```python
from build123d import *

# Parameters (mm, degrees)
SKETCH1_R           = 1.5
BOSS_EXTRUDE1_DEPTH = 3
FILLET1_R           = 0.5


with BuildPart() as part:
    # Sketch1 → Boss-Extrude1 (new body)
    with BuildSketch(Plane.XY):
        with BuildLine():
            ThreePointArc((31, -4), (35, 0), (31, 4))
            Line((31, 4), (11.967993881, 4))
            ThreePointArc((11.967993881, 4), (12.864888434, 4.573115684), (13.63194632, 5.311020574))
            ThreePointArc((13.63194632, 5.311020574), (13.516357561, 5.598658616), (13.394700346, 5.883783021))
            ThreePointArc((13.394700346, 5.883783021), (12.067442445, 5.825370588), (10.794615193, 5.444665539))
            ThreePointArc((10.794615193, 5.444665539), (10.470247132, 6.045), (10.112526268, 6.626078212))
            ThreePointArc((10.112526268, 6.626078212), (11.078640138, 7.538026423), (11.79285574, 8.658259265))
            ThreePointArc((11.79285574, 8.658259265), (11.606759368, 8.906179706), (11.415451897, 9.150101529))
            ThreePointArc((11.415451897, 9.150101529), (10.148537462, 8.750159829), (9.017614465, 8.052995056))
            ThreePointArc((9.017614465, 8.052995056), (8.548920985, 8.548920985), (8.052995056, 9.017614465))
            ThreePointArc((8.052995056, 9.017614465), (8.750159829, 10.148537462), (9.150101529, 11.415451897))
            ThreePointArc((9.150101529, 11.415451897), (8.906179706, 11.606759368), (8.658259265, 11.79285574))
            ThreePointArc((8.658259265, 11.79285574), (7.538026423, 11.078640138), (6.626078212, 10.112526268))
            ThreePointArc((6.626078212, 10.112526268), (6.045, 10.470247132), (5.444665539, 10.794615193))
            ThreePointArc((5.444665539, 10.794615193), (5.825370588, 12.067442445), (5.883783021, 13.394700346))
            ThreePointArc((5.883783021, 13.394700346), (5.598658616, 13.516357561), (5.311020574, 13.63194632))
            ThreePointArc((5.311020574, 13.63194632), (4.413811339, 12.65212943), (3.78298568, 11.482905527))
            ThreePointArc((3.78298568, 11.482905527), (3.129122255, 11.67804324), (2.465291063, 11.835980736))
            ThreePointArc((2.465291063, 11.835980736), (2.503591968, 13.163971168), (2.216494423, 14.461122103))
            ThreePointArc((2.216494423, 14.461122103), (1.909598192, 14.504838322), (1.601844607, 14.542042286))
            ThreePointArc((1.601844607, 14.542042286), (0.988802307, 13.36339701), (0.682088925, 12.070743751))
            ThreePointArc((0.682088925, 12.070743751), (0, 12.09), (-0.682088925, 12.070743751))
            ThreePointArc((-0.682088925, 12.070743751), (-0.988802307, 13.36339701), (-1.601844607, 14.542042286))
            ThreePointArc((-1.601844607, 14.542042286), (-1.909598192, 14.504838322), (-2.216494423, 14.461122103))
            ThreePointArc((-2.216494423, 14.461122103), (-2.503591968, 13.163971168), (-2.465291063, 11.835980736))
            ThreePointArc((-2.465291063, 11.835980736), (-3.129122255, 11.67804324), (-3.78298568, 11.482905527))
            ThreePointArc((-3.78298568, 11.482905527), (-4.413811339, 12.65212943), (-5.311020574, 13.63194632))
            ThreePointArc((-5.311020574, 13.63194632), (-5.598658616, 13.516357561), (-5.883783021, 13.394700346))
            ThreePointArc((-5.883783021, 13.394700346), (-5.825370588, 12.067442445), (-5.444665539, 10.794615193))
            ThreePointArc((-5.444665539, 10.794615193), (-6.045, 10.470247132), (-6.626078212, 10.112526268))
            ThreePointArc((-6.626078212, 10.112526268), (-7.538026423, 11.078640138), (-8.658259265, 11.79285574))
            ThreePointArc((-8.658259265, 11.79285574), (-8.906179706, 11.606759368), (-9.150101529, 11.415451897))
            ThreePointArc((-9.150101529, 11.415451897), (-8.750159829, 10.148537462), (-8.052995056, 9.017614465))
            ThreePointArc((-8.052995056, 9.017614465), (-8.548920985, 8.548920985), (-9.017614465, 8.052995056))
            ThreePointArc((-9.017614465, 8.052995056), (-10.148537462, 8.750159829), (-11.415451897, 9.150101529))
            ThreePointArc((-11.415451897, 9.150101529), (-11.606759368, 8.906179706), (-11.79285574, 8.658259265))
            ThreePointArc((-11.79285574, 8.658259265), (-11.078640138, 7.538026423), (-10.112526268, 6.626078212))
            ThreePointArc((-10.112526268, 6.626078212), (-10.470247132, 6.045), (-10.794615193, 5.444665539))
            ThreePointArc((-10.794615193, 5.444665539), (-12.067442445, 5.825370588), (-13.394700346, 5.883783021))
            ThreePointArc((-13.394700346, 5.883783021), (-13.516357561, 5.598658616), (-13.63194632, 5.311020574))
            ThreePointArc((-13.63194632, 5.311020574), (-12.65212943, 4.413811339), (-11.482905527, 3.78298568))
            ThreePointArc((-11.482905527, 3.78298568), (-11.67804324, 3.129122255), (-11.835980736, 2.465291063))
            ThreePointArc((-11.835980736, 2.465291063), (-13.163971168, 2.503591968), (-14.461122103, 2.216494423))
            ThreePointArc((-14.461122103, 2.216494423), (-14.504838322, 1.909598192), (-14.542042286, 1.601844607))
            ThreePointArc((-14.542042286, 1.601844607), (-13.36339701, 0.988802307), (-12.070743751, 0.682088925))
            ThreePointArc((-12.070743751, 0.682088925), (-12.09, 0), (-12.070743751, -0.682088925))
            ThreePointArc((-12.070743751, -0.682088925), (-13.36339701, -0.988802307), (-14.542042286, -1.601844607))
            ThreePointArc((-14.542042286, -1.601844607), (-14.504838322, -1.909598192), (-14.461122103, -2.216494423))
            ThreePointArc((-14.461122103, -2.216494423), (-13.163971168, -2.503591968), (-11.835980736, -2.465291063))
            ThreePointArc((-11.835980736, -2.465291063), (-11.67804324, -3.129122255), (-11.482905527, -3.78298568))
            ThreePointArc((-11.482905527, -3.78298568), (-12.65212943, -4.413811339), (-13.63194632, -5.311020574))
            ThreePointArc((-13.63194632, -5.311020574), (-13.516357561, -5.598658616), (-13.394700346, -5.883783021))
            ThreePointArc((-13.394700346, -5.883783021), (-12.067442445, -5.825370588), (-10.794615193, -5.444665539))
            ThreePointArc((-10.794615193, -5.444665539), (-10.470247132, -6.045), (-10.112526268, -6.626078212))
            ThreePointArc((-10.112526268, -6.626078212), (-11.078640138, -7.538026423), (-11.79285574, -8.658259265))
            ThreePointArc((-11.79285574, -8.658259265), (-11.606759368, -8.906179706), (-11.415451897, -9.150101529))
            ThreePointArc((-11.415451897, -9.150101529), (-10.148537462, -8.750159829), (-9.017614465, -8.052995056))
            ThreePointArc((-9.017614465, -8.052995056), (-8.548920985, -8.548920985), (-8.052995056, -9.017614465))
            ThreePointArc((-8.052995056, -9.017614465), (-8.750159829, -10.148537462), (-9.150101529, -11.415451897))
            ThreePointArc((-9.150101529, -11.415451897), (-8.906179706, -11.606759368), (-8.658259265, -11.79285574))
            ThreePointArc((-8.658259265, -11.79285574), (-7.538026423, -11.078640138), (-6.626078212, -10.112526268))
            ThreePointArc((-6.626078212, -10.112526268), (-6.045, -10.470247132), (-5.444665539, -10.794615193))
            ThreePointArc((-5.444665539, -10.794615193), (-5.825370588, -12.067442445), (-5.883783021, -13.394700346))
            ThreePointArc((-5.883783021, -13.394700346), (-5.598658616, -13.516357561), (-5.311020574, -13.63194632))
            ThreePointArc((-5.311020574, -13.63194632), (-4.413811339, -12.65212943), (-3.78298568, -11.482905527))
            ThreePointArc((-3.78298568, -11.482905527), (-3.129122255, -11.67804324), (-2.465291063, -11.835980736))
            ThreePointArc((-2.465291063, -11.835980736), (-2.503591968, -13.163971168), (-2.216494423, -14.461122103))
            ThreePointArc((-2.216494423, -14.461122103), (-1.909598192, -14.504838322), (-1.601844607, -14.542042286))
            ThreePointArc((-1.601844607, -14.542042286), (-0.988802307, -13.36339701), (-0.682088925, -12.070743751))
            ThreePointArc((-0.682088925, -12.070743751), (0, -12.09), (0.682088925, -12.070743751))
            ThreePointArc((0.682088925, -12.070743751), (0.988802307, -13.36339701), (1.601844607, -14.542042286))
            ThreePointArc((1.601844607, -14.542042286), (1.909598192, -14.504838322), (2.216494423, -14.461122103))
            ThreePointArc((2.216494423, -14.461122103), (2.503591968, -13.163971168), (2.465291063, -11.835980736))
            ThreePointArc((2.465291063, -11.835980736), (3.129122255, -11.67804324), (3.78298568, -11.482905527))
            ThreePointArc((3.78298568, -11.482905527), (4.413811339, -12.65212943), (5.311020574, -13.63194632))
            ThreePointArc((5.311020574, -13.63194632), (5.598658616, -13.516357561), (5.883783021, -13.394700346))
            ThreePointArc((5.883783021, -13.394700346), (5.825370588, -12.067442445), (5.444665539, -10.794615193))
            ThreePointArc((5.444665539, -10.794615193), (6.045, -10.470247132), (6.626078212, -10.112526268))
            ThreePointArc((6.626078212, -10.112526268), (7.538026423, -11.078640138), (8.658259265, -11.79285574))
            ThreePointArc((8.658259265, -11.79285574), (8.906179706, -11.606759368), (9.150101529, -11.415451897))
            ThreePointArc((9.150101529, -11.415451897), (8.750159829, -10.148537462), (8.052995056, -9.017614465))
            ThreePointArc((8.052995056, -9.017614465), (8.548920985, -8.548920985), (9.017614465, -8.052995056))
            ThreePointArc((9.017614465, -8.052995056), (10.148537462, -8.750159829), (11.415451897, -9.150101529))
            ThreePointArc((11.415451897, -9.150101529), (11.606759368, -8.906179706), (11.79285574, -8.658259265))
            ThreePointArc((11.79285574, -8.658259265), (11.078640138, -7.538026423), (10.112526268, -6.626078212))
            ThreePointArc((10.112526268, -6.626078212), (10.470247132, -6.045), (10.794615193, -5.444665539))
            ThreePointArc((10.794615193, -5.444665539), (12.067442445, -5.825370588), (13.394700346, -5.883783021))
            ThreePointArc((13.394700346, -5.883783021), (13.516357561, -5.598658616), (13.63194632, -5.311020574))
            ThreePointArc((13.63194632, -5.311020574), (12.864888434, -4.573115684), (11.967993881, -4))
            Line((11.967993881, -4), (31, -4))
        make_face()
        Circle(SKETCH1_R, mode=Mode.SUBTRACT)
        with Locations((31, 0)):
            Circle(SKETCH1_R, mode=Mode.SUBTRACT)
    extrude(amount=-BOSS_EXTRUDE1_DEPTH)

    # Fillet1
    fillet1_edges = [part.edges().sort_by_distance(p)[0] for p in [
        (-1.5, 0, -3),
        (-1.5, 0, 0),
        (29.5, 0, 0),
        (29.5, 0, -3),
    ]]
    fillet(fillet1_edges, radius=FILLET1_R)


solid = part.part
```
Build history of the part. All positions in model axes, mm. A direction names the side the tool comes from. Coordinates: 2 decimals unless noted, no trailing zeros. Order: outer loops, then holes, each group sorted by start corner. A loop starts at its lowest first (then second) coordinate and runs counter-clockwise, first axis right, second up. Notation, with made-up numbers: (2, 57) -> (38, 57) arc R25 ccw to (38, 94) -> close; hole circle Ø3 at (12, -17.75). An arc over 180 degrees is marked (long way). Answer in a Markdown table with one row per item. Add a question column.
Q1. Drop flat-ended pins along their axis: pin 1 (0.9 mm diameter, centred on x = 22, z = -1.5, fed in from +Y); pin 2 (1.5 mm diameter, centred on x = 11.5, z = -1, fed in from +Y); pin 3 (2.5 mm diameter, centred on x = 0, y = 0, fed in from +Z) (1 decimal); pin 4 (5 mm diameter, centred on x = 31, y = 0, fed in from -Z). Give the stop position or say it passes through.
Q2. Which spindle directions (+Z, -Z, +X, -X, +Y, -Y) get a long thin tool onto all of the face, cutting with end or side? Do faces 1 (the face through (-4.425, -12.667, -1.479)), 2 (the face through (10.475, 6.037, -1.479)), 3 (the face through (-12.09, 0.01, -1.48)), 4 (the face through (4.425, 12.667, -1.479)). Say none if no direction does.
Q3. Wall check: line 1 along Y through (x, z) = (31, -1.4); line 2 along X through (y, z) = (1.25, -0.3); line 3 along Y through (x, z) = (21.5, -1.6). Give the ranges that are in metal, low to high. Write a range as [from, to].
Q4. Band-saw the part on B-B, the plane x = 0. List the corners of the cut face in (y, z), then the cut area to 3 significant figures.
Q5. Mould opens along X. For faces 5 (the face through (-3.138, -11.676, -1.479)), 6 (the face through (-12.667, 4.425, -1.479)) say: +X half, -X half, draft (parallel to the pull), parting line (faces both ways), or undercut.
Q6. Band-saw the part on A-A, the plane y = 0. List the corners of the cut face in (x, z).
Answers follow:
| question | item | result |
|---|---|---|
| 1 | pin 1 | y = 4 |
| 1 | pin 2 | y = 9.15 |
| 1 | pin 3 | through |
| 1 | pin 4 | z = -3 |
| 2 | face 1 | +Z, -Z, -Y |
| 2 | face 2 | +Z, -Z |
| 2 | face 3 | +Z, -Z, -X |
| 2 | face 4 | +Z, -Z, +Y |
| 3 | line 1 | [-4, -1.5], [1.5, 4] |
| 3 | line 2 | [-13.95, -0.9], [0.9, 30.1], [31.9, 34.8] |
| 3 | line 3 | [-4, 4] |
| 4 | outline | (-12.09, -3) -> (-2, -3) arc R0.5 ccw to (-1.5, -2.5) -> (-1.5, -0.5) arc R0.5 ccw to (-2, 0) -> (-12.09, 0) -> close; (1.5, -2.5) arc R0.5 ccw to (2, -3) -> (12.09, -3) -> (12.09, 0) -> (2, 0) arc R0.5 ccw to (1.5, -0.5) -> close |
| 4 | area | 63.3 mm^2 |
| 5 | face 5 | undercut |
| 5 | face 6 | -X half |
| 6 | outline | (-12.09, -3) -> (-2, -3) arc R0.5 ccw to (-1.5, -2.5) -> (-1.5, -0.5) arc R0.5 ccw to (-2, 0) -> (-12.09, 0) -> close; (1.5, -2.5) arc R0.5 ccw to (2, -3) -> (29, -3) arc R0.5 ccw to (29.5, -2.5) -> (29.5, -0.5) arc R0.5 ccw to (29, 0) -> (2, 0) arc R0.5 ccw to (1.5, -0.5) -> close; (32.5, -2.5) arc R0.5 ccw to (33, -3) -> (35, -3) -> (35, 0) -> (33, 0) arc R0.5 ccw to (32.5, -0.5) -> close |
